Check sheet for the modelled part. Datum: model origin and axes. Units: mm. Give positions to 0.01 mm unless a question says otherwise; leave off trailing zeros.
Item 1: Gauge pin test, flat ends, axial feed: P1, Ø10, axis at x = 20.5, z = 16.5, coming from the -Y side; P2, Ø12, axis at x = -9.5, y = 7.5, coming from the -Z side; P3, Ø2, axis at y = -14, z = 13.5, coming from the +X side; P4, Ø1, axis at x = -22, y = 10, coming from the +Z side. Record the tip position at first contact, or that the pin passes through.
Item 2: Release check for a two-part mould opening along X. For faces 1 (the flat face through (16, -16, 0)), 2 (the cylindrical face through (21.199, 6.676, 15.256)) record: released by +X, released by -X, zero draft, split by the parting line, or undercut.
Item 3: Material ranges on line 1 along X through (y, z) = (0, 21) (3 decimals); line 2 along X through (y, z) = (-7.5, 11), recorded low to high.
from build123d import *

# Parameters (mm, degrees)
F0_R     = 38.1
F1_DEPTH = 38.1
F2_R     = 38.09999
F3_R     = 22.225
F4_DEPTH = 151.384


# Not quite as in the source:
# - a fillet or chamfer is up to 0.001 mm smaller than in the source, because OpenCascade refuses the exact size


with BuildPart() as f1:
    # F0 (on Top) → F1 (new body)
    with BuildSketch(Plane.XY):
        Circle(F0_R)
    extrude(amount=F1_DEPTH)

    # F2 (radius 38.1 in the source; OpenCascade refuses exactly that, so slightly less here)
    f2_edges = [f1.edges().sort_by_distance(p)[0] for p in [
        (-38.1, 0, 38.1),
    ]]
    fillet(f2_edges, radius=F2_R)

    # F3 (on Top) → F4 (cut)
    with BuildSketch(Plane.XY):
        Circle(F3_R)
    extrude(amount=F4_DEPTH, mode=Mode.SUBTRACT)


solid = f1.part
Report:
1. P1: stops at y = -31.58
1. P2: passes through
1. P3: stops at x = 33.34
1. P4: stops at z = 29.86
2. face 1: zero draft
2. face 2: undercut
3. line 1: x = -31.79 to -22.225, 22.225 to 31.79
3. line 2: x = -35.7 to -20.92, 20.92 to 35.7
